Verification items for the finished model (mm, model axes). Round coordinates to 2 decimals unless told otherwise and drop trailing zeros. Write each loop counter-clockwise with the first axis right and the second up, starting at its lowest first coordinate (ties: lowest second). Pieces come first, ordered by that corner, then holes.
from build123d import *

# Parameters (mm, degrees)
SKETCH1_W           = 25.4
SKETCH1_H           = 25.4
BOSS_EXTRUDE1_DEPTH = 5


with BuildPart() as part:
    # Sketch1 → Boss-Extrude1 (new body)
    with BuildSketch(Plane(origin=(0, 0, 0), x_dir=(1, 0, 0), z_dir=(0, 1, 0))):
        with BuildLine():
            Line((110, 155.4), (110, 175.11258305))
            ThreePointArc((110, 175.11258305), (0, 187.619127597), (-110, 175.11258305))
            Line((-110, 175.11258305), (-110, 155.4))
            Line((-110, 155.4), (-115, 155.4))
            Line((-115, 155.4), (-115, 173.933099678))
            ThreePointArc((-115, 173.933099678), (-137.944531709, 167.801332887), (-160.565, 160.565))
            ThreePointArc((-160.565, 160.565), (-167.801332887, 137.944531709), (-173.933099678, 115))
            Line((-173.933099678, 115), (-155.4, 115))
            Line((-155.4, 115), (-155.4, 110))
            Line((-155.4, 110), (-175.11258305, 110))
            ThreePointArc((-175.11258305, 110), (-187.619127597, 0), (-175.11258305, -110))
            Line((-175.11258305, -110), (-155.4, -110))
            Line((-155.4, -110), (-155.4, -115))
            Line((-155.4, -115), (-173.933099678, -115))
            ThreePointArc((-173.933099678, -115), (-167.801332887, -137.944531709), (-160.565, -160.565))
            ThreePointArc((-160.565, -160.565), (-137.944531709, -167.801332887), (-115, -173.933099678))
            Line((-115, -173.933099678), (-115, -155.4))
            Line((-115, -155.4), (-110, -155.4))
            Line((-110, -155.4), (-110, -175.11258305))
            ThreePointArc((-110, -175.11258305), (0, -187.619127597), (110, -175.11258305))
            Line((110, -175.11258305), (110, -155.4))
            Line((110, -155.4), (115, -155.4))
            Line((115, -155.4), (115, -173.933099678))
            ThreePointArc((115, -173.933099678), (137.944531709, -167.801332887), (160.565, -160.565))
            ThreePointArc((160.565, -160.565), (167.801332887, -137.944531709), (173.933099678, -115))
            Line((173.933099678, -115), (155.4, -115))
            Line((155.4, -115), (155.4, -110))
            Line((155.4, -110), (175.11258305, -110))
            ThreePointArc((175.11258305, -110), (187.619127597, 0), (175.11258305, 110))
            Line((175.11258305, 110), (155.4, 110))
            Line((155.4, 110), (155.4, 115))
            Line((155.4, 115), (173.933099678, 115))
            ThreePointArc((173.933099678, 115), (167.801332887, 137.944531709), (160.565, 160.565))
            ThreePointArc((160.565, 160.565), (137.944531709, 167.801332887), (115, 173.933099678))
            Line((115, 173.933099678), (115, 155.4))
            Line((115, 155.4), (110, 155.4))
        make_face()
        with Locations((-127.7, 127.7)):
            Rectangle(SKETCH1_W, SKETCH1_H, mode=Mode.SUBTRACT)
        with Locations((127.7, 127.7)):
            Rectangle(SKETCH1_W, SKETCH1_H, mode=Mode.SUBTRACT)
        with Locations((127.7, -127.7)):
            Rectangle(SKETCH1_W, SKETCH1_H, mode=Mode.SUBTRACT)
        with Locations((-127.7, -127.7)):
            Rectangle(SKETCH1_W, SKETCH1_H, mode=Mode.SUBTRACT)
    extrude(amount=BOSS_EXTRUDE1_DEPTH)


solid = part.part
Q1. Sectioned sample at C-C (x = -60.5). Enter the section's corners in (y, z), plus the area to 3 significant figures.
Recorded:
outline: (0, -183.87) - (5, -183.87) - (5, 183.87) - (0, 183.87) - close
area: 1,840 mm2
Q2. Material ranges on line 1 along X through (y, z) = (4.15, 131.5); line 2 along X through (y, z) = (2.8, 122.5); line 3 along Z through (x, y) = (140, 4.6), recorded low to high.
Recorded:
line 1: x = -169.64 to -140.4, -115 to 115, 140.4 to 169.64
line 2: x = -172.06 to -140.4, -115 to 115, 140.4 to 172.06
line 3: z = -167.19 to -140.4, -115 to 115, 140.4 to 167.19
Q3. Sectioned sample at A-A (y = 2.8). Give the number of separate pieces and of enclosed holes in the cut face, plus the area to 3 significant figures.
Recorded:
separate pieces: 1
enclosed holes: 4
area: 123,000 mm2
Q4. Sectioned sample at B-B (z = -102.5). Enter the section's corners in (x, y).
Recorded:
outline: (-176.78, 0) - (176.78, 0) - (176.78, 5) - (-176.78, 5) - close
Q5. Depth check by flat-ended pin: P1, Ø2.5, axis at y = 3, z = -124, coming from the -X side; P2, Ø1.5, axis at x = -127.5, y = 3.5, coming from the -Z side; P3, Ø3, axis at y = 1, z = -138, coming from the -X side; P4, Ø10, axis at x = 139.5, z = 148.5, coming from the -Y side. Enter the tip coordinate at first touch or a pass-through.
Recorded:
P1: stops at x = -171.99
P2: stops at z = -170.94
P3: stops at x = -168.22
P4: stops at y = 0
